```python
from build123d import *

# Parameters (mm, degrees)
F0_R     = 3.175
F1_DEPTH = 25.4


with BuildPart() as f1:
    # F0 (on Front) → F1 (new body)
    with BuildSketch(Plane.XZ):
        with BuildLine():
            ThreePointArc((3.175, 0), (-2.2450640303, -2.2450640303), (0, 3.175))
            Line((0, 3.175), (0, 9.525))
            ThreePointArc((0, 9.525), (-9.525, 0), (0, -9.525))
            Line((0, -9.525), (0.6773435479, -9.500885786))
            ThreePointArc((0.6773435479, -9.500885786), (6.9705567315, -6.4912990883), (9.525, 0))
            Line((9.525, 0), (3.175, 0))
        make_face()
        with BuildLine():
            Line((0, 9.525), (0, 3.175))
            ThreePointArc((0, 3.175), (2.2450640303, 2.2450640303), (3.175, 0))
            Line((3.175, 0), (9.525, 0))
            ThreePointArc((9.525, 0), (6.7351920908, 6.7351920908), (0, 9.525))
        make_face()
        with BuildLine():
            Line((0, 47.625), (0, 9.525))
            ThreePointArc((0, 9.525), (6.7351920908, 6.7351920908), (9.525, 0))
            Line((9.525, 0), (36.5125, 0))
            ThreePointArc((36.5125, 0), (40.830361875, 7.0641436915), (49.0862640553, 6.442744901))
            Line((49.0862640553, 6.442744901), (16.5675029115, 29.8435726117))
            ThreePointArc((16.5675029115, 29.8435726117), (13.9631116964, 33.0299588598), (13.3008358668, 37.0916459046))
            Line((13.3008358668, 37.0916459046), (15.7954255641, 61.9125))
            ThreePointArc((15.7954255641, 61.9125), (10.6492737428, 51.7267849017), (0, 47.625))
        make_face()
        with BuildLine():
            Line((36.5125, 0), (9.525, 0))
            ThreePointArc((9.525, 0), (6.9705567315, -6.4912990883), (0.6773435479, -9.500885786))
            Line((0.6773435479, -9.500885786), (27.1872243516, -8.5571033561))
            Line((27.1872243516, -8.5571033561), (44.7324052746, -7.9324746146))
            ThreePointArc((44.7324052746, -7.9324746146), (38.9380895153, -5.7116327839), (36.5125, 0))
        make_face()
        with BuildLine():
            ThreePointArc((-15.7954255641, 61.9125), (-10.6492737428, 51.7267849017), (0, 47.625))
            Line((0, 47.625), (0, 60.325))
            ThreePointArc((0, 60.325), (-3.175, 63.5), (0, 66.675))
            Line((0, 66.675), (0, 79.375))
            ThreePointArc((0, 79.375), (-10.5003255158, 75.40625), (-15.7504882737, 65.484375))
            ThreePointArc((-15.7504882737, 65.484375), (-15.8737438155, 63.6997054867), (-15.7954255641, 61.9125))
        make_face()
        with BuildLine():
            Line((0, 60.325), (0, 47.625))
            ThreePointArc((0, 47.625), (10.6492737428, 51.7267849017), (15.7954255641, 61.9125))
            ThreePointArc((15.7954255641, 61.9125), (15.8550939106, 62.7052534459), (15.875, 63.5))
            ThreePointArc((15.875, 63.5), (15.8438414904, 64.4941387366), (15.7504882737, 65.484375))
            ThreePointArc((15.7504882737, 65.484375), (10.5003255158, 75.40625), (0, 79.375))
            Line((0, 79.375), (0, 66.675))
            ThreePointArc((0, 66.675), (2.2450640303, 65.7450640303), (3.175, 63.5))
            ThreePointArc((3.175, 63.5), (2.2450640303, 61.2549359697), (0, 60.325))
        make_face()
        with BuildLine():
            Line((0.6773435479, -9.500885786), (0, -9.525))
            ThreePointArc((0, -9.525), (0.3388863295, -9.5189695375), (0.6773435479, -9.500885786))
        make_face()
        with BuildLine():
            ThreePointArc((49.0862640553, 6.442744901), (40.830361875, 7.0641436915), (36.5125, 0))
            ThreePointArc((36.5125, 0), (38.9380895153, -5.7116327839), (44.7324052746, -7.9324746146))
            ThreePointArc((44.7324052746, -7.9324746146), (50.1616327839, -5.5119104847), (52.3875, 0))
            ThreePointArc((52.3875, 0), (51.5141436915, 3.619638125), (49.0862640553, 6.442744901))
        make_face()
        with BuildLine():
            ThreePointArc((47.625, 0), (44.45, -3.175), (41.275, 0))
            ThreePointArc((41.275, 0), (44.45, 3.175), (47.625, 0))
        make_face(mode=Mode.SUBTRACT)
        with BuildLine():
            Line((-9.4502929642, 115.490625), (-15.7504882737, 65.484375))
            ThreePointArc((-15.7504882737, 65.484375), (-10.5003255158, 75.40625), (0, 79.375))
            Line((0, 79.375), (0, 104.775))
            ThreePointArc((0, 104.775), (-7.14375, 107.9998046905), (-9.4502929642, 115.490625))
        make_face()
        with Locations((-5.8028255589, 100.0252)):
            Circle(F0_R, mode=Mode.SUBTRACT)
        with BuildLine():
            Line((0, 104.775), (0, 79.375))
            ThreePointArc((0, 79.375), (10.5003255158, 75.40625), (15.7504882737, 65.484375))
            Line((15.7504882737, 65.484375), (9.4502929642, 115.490625))
            ThreePointArc((9.4502929642, 115.490625), (9.5063048942, 114.896483242), (9.525, 114.3))
            ThreePointArc((9.525, 114.3), (6.7351920908, 107.5648079092), (0, 104.775))
        make_face()
        with BuildLine():
            ThreePointArc((9.4502929642, 115.490625), (0, 123.825), (-9.4502929642, 115.490625))
            ThreePointArc((-9.4502929642, 115.490625), (-7.14375, 107.9998046905), (0, 104.775))
            ThreePointArc((0, 104.775), (6.7351920908, 107.5648079092), (9.525, 114.3))
            ThreePointArc((9.525, 114.3), (9.5063048942, 114.896483242), (9.4502929642, 115.490625))
        make_face()
        with BuildLine():
            ThreePointArc((3.175, 114.3), (2.2450640303, 112.0549359697), (0, 111.125))
            ThreePointArc((0, 111.125), (-2.2450640303, 116.5450640303), (3.175, 114.3))
        make_face(mode=Mode.SUBTRACT)
    extrude(amount=F1_DEPTH)


solid = f1.part
```
Could you check a few things on this model? Use its own coordinates, in mm. A direction names the side the tool comes from. Round coordinates to 2 decimals unless told otherwise and drop trailing zeros. Loops run counter-clockwise (first coordinate to the right, second up) from the corner with the lowest first, then second, coordinate; pieces in that order, holes last.
Q1. I want a section at A-A (y = -12). Give the number of separate pieces and of enclosed holes in the cut face, and give its area (3 significant figures).
Q2. I want a section at B-B (z = 53.5). Write out the boundary of the cut face in (x, y), and give its area (3 significant figures).
Q3. Please list where these lines run through material, in increasing order: L1, parallel to Z at x = -1, y = -12.5; L2, parallel to Z at x = 2.5, y = -8.75; L3, parallel to X at y = -23.5, z = 63.
Q4. For P1, Ø6, axis at x = 37, y = -5.5, coming from the -Z side; P2, Ø10, axis at y = -3, z = 29.5, coming from the +X side; P3, Ø6, axis at x = -4, y = -13, coming from the -Z side, each with a flat end and sliding along its axis, tell me the tip position at first contact or that it passes through.
Q5. Thinking about a two-plate mould opening in Z: for faces 1 (the cylindrical face through (0.193, -12.522, 123.823)), 2 (the flat face through (10, 0, 43)), 3 (the cylindrical face through (41.52, -12.52, -1.22)), which applies, pulls with the +Z half, pulls with the -Z half, needs draft (parallel to the pull), parting line crosses it, or undercut?
Q6. On a 3-axis mill with a long thin cutter (end or side, diameter ignored), from which of +Z, -Z, +X, -X, +Y, -Y can I reach the whole of each face in a straight line? I mean faces 4 (the flat face through (0, -13, 29)), 5 (the flat face through (-12.556, -12.522, 90.838)), 6 (the flat face through (14.53, -12.52, 49.33)). Say none if no direction works.
Answer below:
1. separate pieces: 1
1. enclosed holes: 5
1. area: 3,650 mm2
2. outline: (-12.33, -25.4) - (14.95, -25.4) - (14.95, 0) - (-12.33, 0) - close
2. area: 693 mm2
3. L1: z = -9.47 to -3.01, 3.01 to 9.47, 47.66 to 60.49, 66.51 to 111.29, 117.31 to 123.77
3. L2: z = -9.44 to -1.96, 1.96 to 61.54, 65.46 to 112.34, 116.26 to 123.49
3. L3: x = -15.87 to -3.14, 3.14 to 15.87
4. P1: stops at z = -8.31
4. P2: stops at x = 23.99
4. P3: stops at z = -9.47
5. face 1: pulls with the +Z half
5. face 2: needs draft
5. face 3: undercut
6. face 4: -X, +Y, -Y
6. face 5: +Z, -X, +Y, -Y
6. face 6: +X, +Y, -Y
